```python
from build123d import *

# Parameters (mm, degrees)
BOSS_EXTRUDE1_DEPTH   = 2
BOSS_EXTRUDE1_2_DEPTH = 2
BOSS_EXTRUDE1_3_DEPTH = 2
SKETCH3_W             = 15
SKETCH3_H             = 6
BOSS_EXTRUDE2_DEPTH   = 2


with BuildPart() as part:
    # Sketch2 → Boss-Extrude1 (new body)
    with BuildSketch(Plane.XY):
        with BuildLine():
            Line((11.971746688, 19.734053644), (13.156348071, 19.734053669))
            ThreePointArc((13.156348071, 19.734053669), (13.179525443, 19.744291413), (13.193365664, 19.765515226))
            ThreePointArc((13.193365664, 19.765515226), (13.19739915, 19.821201025), (13.188063691, 19.8762467))
            ThreePointArc((13.188063691, 19.8762467), (13.111547426, 20.044582448), (13.014440765, 20.20194178))
            add(Edge.make_bspline(
                [(13.014440765, 20.20194178), (12.484950193, 21.013504257), (11.291530639, 21.013504258)],
                knots=[0.342748392, 0.342748392, 0.342748392, 1.381331673, 1.381331673, 1.381331673], degree=2, weights=[1, 0.868170932, 1]))
            Line((11.291530639, 21.013504258), (11.173022933, 21.013504277))
            add(Edge.make_bspline(
                [(11.173022933, 21.013504277), (9.165862366, 21.013504277), (9.16586234, 19.429763689)],
                knots=[4.81203319, 4.81203319, 4.81203319, 6.344970319, 6.344970319, 6.344970319], degree=2, weights=[1, 0.720364545, 1]))
            Line((9.16586234, 19.429763689), (9.165862348, 19.265041834))
            add(Edge.make_bspline(
                [(9.165862348, 19.265041834), (9.165862348, 17.681301204), (11.173022971, 17.681301277)],
                knots=[3.079807634, 3.079807634, 3.079807634, 4.612744788, 4.612744788, 4.612744788], degree=2, weights=[1, 0.720364536, 1]))
            Line((11.173022971, 17.681301277), (11.291530595, 17.681301231))
            add(Edge.make_bspline(
                [(11.291530595, 17.681301231), (12.48495018, 17.681301231), (13.014440765, 18.492863728)],
                knots=[1.760260959, 1.760260959, 1.760260959, 2.798844261, 2.798844261, 2.798844261], degree=2, weights=[1, 0.868170926, 1]))
            ThreePointArc((13.014440765, 18.492863728), (13.107795315, 18.64362681), (13.182053506, 18.804655688))
            ThreePointArc((13.182053506, 18.804655688), (13.196728173, 18.865824439), (13.194497656, 18.928689268))
            ThreePointArc((13.194497656, 18.928689268), (13.179302023, 18.955174053), (13.150618481, 18.965643321))
            Line((13.150618481, 18.965643321), (11.971746647, 18.965643321))
            ThreePointArc((11.971746647, 18.965643321), (11.923939268, 18.950452436), (11.893668965, 18.91045222))
            add(Edge.make_bspline(
                [(11.265198612, 18.440979368), (11.727360525, 18.440524679), (11.893668965, 18.91045222)],
                knots=[5.955155363, 5.955155363, 5.955155363, 7.020735544, 7.020735544, 7.020735544], degree=2, weights=[1, 0.86139323, 1]))
            add(Edge.make_bspline(
                [(11.189511072, 20.254442875), (10.402055714, 20.214623084), (10.44001251, 19.305183226), (10.477969307, 18.395743368), (11.265198612, 18.440979368)],
                knots=[3.181025595, 3.181025595, 3.181025595, 4.754799698, 4.754799698, 6.328573801, 6.328573801, 6.328573801], degree=2, weights=[1, 0.706053195, 1, 0.706053195, 1]))
            add(Edge.make_bspline(
                [(11.893668965, 19.789244771), (11.708556533, 20.312305593), (11.189511072, 20.254442875)],
                knots=[2.404042417, 2.404042417, 2.404042417, 3.565685694, 3.565685694, 3.565685694], degree=2, weights=[1, 0.83601209, 1]))
            ThreePointArc((11.893668965, 19.789244771), (11.923939288, 19.749244541), (11.971746688, 19.734053644))
        make_face()
    extrude(amount=BOSS_EXTRUDE1_DEPTH)



with BuildPart() as body_2:
    # Sketch2 → Boss-Extrude1 2 (new body)
    with BuildSketch(Plane.XY):
        with BuildLine():
            Line((7.784019348, 19.734053644), (8.968620799, 19.734053669))
            ThreePointArc((8.968620799, 19.734053669), (8.99179817, 19.744291413), (9.005638392, 19.765515226))
            ThreePointArc((9.005638392, 19.765515226), (9.009671877, 19.821201025), (9.000336418, 19.8762467))
            ThreePointArc((9.000336418, 19.8762467), (8.923820153, 20.044582448), (8.826713493, 20.20194178))
            add(Edge.make_bspline(
                [(8.826713493, 20.20194178), (8.29722292, 21.013504257), (7.103803365, 21.013504258)],
                knots=[0.342748392, 0.342748392, 0.342748392, 1.381331673, 1.381331673, 1.381331673], degree=2, weights=[1, 0.868170932, 1]))
            Line((7.103803365, 21.013504258), (6.98529566, 21.013504277))
            add(Edge.make_bspline(
                [(6.98529566, 21.013504277), (4.978135095, 21.013504277), (4.978135132, 19.429763689)],
                knots=[4.81203319, 4.81203319, 4.81203319, 6.344970317, 6.344970317, 6.344970317], degree=2, weights=[1, 0.720364545, 1]))
            Line((4.978135132, 19.429763689), (4.978135076, 19.265041834))
            add(Edge.make_bspline(
                [(4.978135076, 19.265041834), (4.978135076, 17.681301205), (6.985295697, 17.681301277)],
                knots=[3.079807634, 3.079807634, 3.079807634, 4.612744788, 4.612744788, 4.612744788], degree=2, weights=[1, 0.720364536, 1]))
            Line((6.985295697, 17.681301277), (7.103803322, 17.681301231))
            add(Edge.make_bspline(
                [(7.103803322, 17.681301231), (8.297222907, 17.681301231), (8.826713493, 18.492863728)],
                knots=[4.901853612, 4.901853612, 4.901853612, 5.940436915, 5.940436915, 5.940436915], degree=2, weights=[1, 0.868170926, 1]))
            ThreePointArc((8.826713493, 18.492863728), (8.920068042, 18.64362681), (8.994326233, 18.804655688))
            ThreePointArc((8.994326233, 18.804655688), (9.009000901, 18.865824439), (9.006770384, 18.928689268))
            ThreePointArc((9.006770384, 18.928689268), (8.99157475, 18.955174054), (8.962891207, 18.965643321))
            Line((8.962891207, 18.965643321), (7.784019375, 18.965643321))
            ThreePointArc((7.784019375, 18.965643321), (7.736211995, 18.950452436), (7.705941692, 18.91045222))
            add(Edge.make_bspline(
                [(7.07747134, 18.440979368), (7.539633252, 18.440524679), (7.705941692, 18.91045222)],
                knots=[5.955155363, 5.955155363, 5.955155363, 7.020735544, 7.020735544, 7.020735544], degree=2, weights=[1, 0.86139323, 1]))
            add(Edge.make_bspline(
                [(7.0017838, 20.254442875), (6.214328441, 20.214623084), (6.252285238, 19.305183226), (6.290242034, 18.395743368), (7.07747134, 18.440979368)],
                knots=[3.181025595, 3.181025595, 3.181025595, 4.754799698, 4.754799698, 6.328573801, 6.328573801, 6.328573801], degree=2, weights=[1, 0.706053195, 1, 0.706053195, 1]))
            add(Edge.make_bspline(
                [(7.705941692, 19.78924477), (7.520829261, 20.312305593), (7.0017838, 20.254442875)],
                knots=[2.404042417, 2.404042417, 2.404042417, 3.565685694, 3.565685694, 3.565685694], degree=2, weights=[1, 0.83601209, 1]))
            ThreePointArc((7.705941692, 19.78924477), (7.736211988, 19.74924456), (7.784019348, 19.734053644))
        make_face()
    extrude(amount=BOSS_EXTRUDE1_2_DEPTH)


with BuildPart() as body_3:
    # Sketch2 → Boss-Extrude1 3 (new body)
    with BuildSketch(Plane.XY):
        with BuildLine():
            Line((16.159473961, 19.734053644), (17.344075345, 19.734053669))
            ThreePointArc((17.344075345, 19.734053669), (17.367252716, 19.744291413), (17.381092938, 19.765515226))
            ThreePointArc((17.381092938, 19.765515226), (17.385126423, 19.821201025), (17.375790964, 19.8762467))
            ThreePointArc((17.375790964, 19.8762467), (17.2992747, 20.044582448), (17.202168039, 20.20194178))
            add(Edge.make_bspline(
                [(17.202168039, 20.20194178), (16.672677467, 21.013504257), (15.479257913, 21.013504258)],
                knots=[0.342748392, 0.342748392, 0.342748392, 1.381331673, 1.381331673, 1.381331673], degree=2, weights=[1, 0.868170932, 1]))
            Line((15.479257913, 21.013504258), (15.360750206, 21.013504277))
            add(Edge.make_bspline(
                [(15.360750206, 21.013504277), (13.353589639, 21.013504277), (13.353589613, 19.429763689)],
                knots=[4.81203319, 4.81203319, 4.81203319, 6.344970319, 6.344970319, 6.344970319], degree=2, weights=[1, 0.720364545, 1]))
            Line((13.353589613, 19.429763689), (13.353589622, 19.265041834))
            add(Edge.make_bspline(
                [(13.353589622, 19.265041834), (13.353589622, 17.681301204), (15.360750245, 17.681301277)],
                knots=[3.079807634, 3.079807634, 3.079807634, 4.612744788, 4.612744788, 4.612744788], degree=2, weights=[1, 0.720364536, 1]))
            Line((15.360750245, 17.681301277), (15.479257869, 17.681301231))
            add(Edge.make_bspline(
                [(15.479257869, 17.681301231), (16.672677453, 17.681301231), (17.202168039, 18.492863728)],
                knots=[1.760260959, 1.760260959, 1.760260959, 2.798844261, 2.798844261, 2.798844261], degree=2, weights=[1, 0.868170926, 1]))
            ThreePointArc((17.202168039, 18.492863728), (17.295522588, 18.64362681), (17.369780779, 18.804655688))
            ThreePointArc((17.369780779, 18.804655688), (17.384455447, 18.865824439), (17.38222493, 18.928689268))
            ThreePointArc((17.38222493, 18.928689268), (17.367029296, 18.955174053), (17.338345755, 18.965643321))
            Line((17.338345755, 18.965643321), (16.159473921, 18.965643321))
            ThreePointArc((16.159473921, 18.965643321), (16.111666541, 18.950452436), (16.081396238, 18.91045222))
            add(Edge.make_bspline(
                [(15.452925886, 18.440979368), (15.915087798, 18.440524679), (16.081396238, 18.91045222)],
                knots=[5.955155363, 5.955155363, 5.955155363, 7.020735544, 7.020735544, 7.020735544], degree=2, weights=[1, 0.86139323, 1]))
            add(Edge.make_bspline(
                [(15.377238346, 20.254442875), (14.589782987, 20.214623084), (14.627739784, 19.305183226), (14.665696581, 18.395743368), (15.452925886, 18.440979368)],
                knots=[3.181025595, 3.181025595, 3.181025595, 4.754799698, 4.754799698, 6.328573801, 6.328573801, 6.328573801], degree=2, weights=[1, 0.706053195, 1, 0.706053195, 1]))
            add(Edge.make_bspline(
                [(16.081396238, 19.789244771), (15.896283807, 20.312305593), (15.377238346, 20.254442875)],
                knots=[2.404042417, 2.404042417, 2.404042417, 3.565685694, 3.565685694, 3.565685694], degree=2, weights=[1, 0.83601209, 1]))
            ThreePointArc((16.081396238, 19.789244771), (16.111666561, 19.749244541), (16.159473961, 19.734053644))
        make_face()
    extrude(amount=BOSS_EXTRUDE1_3_DEPTH)


with BuildPart() as part_1:
    add(part.part)

    add(body_2.part)  # Boss-Extrude2 merges body 2

    add(body_3.part)  # Boss-Extrude2 merges body 3
    # Sketch3 → Boss-Extrude2 (add)
    with BuildSketch(Plane(origin=(0, 0, 0), x_dir=(-1, 0, 0), z_dir=(0, 0, -1))):
        with Locations((-11.178135076, 19.347504277)):
            Rectangle(SKETCH3_W, SKETCH3_H)
    extrude(amount=BOSS_EXTRUDE2_DEPTH)


solid = part_1.part
```
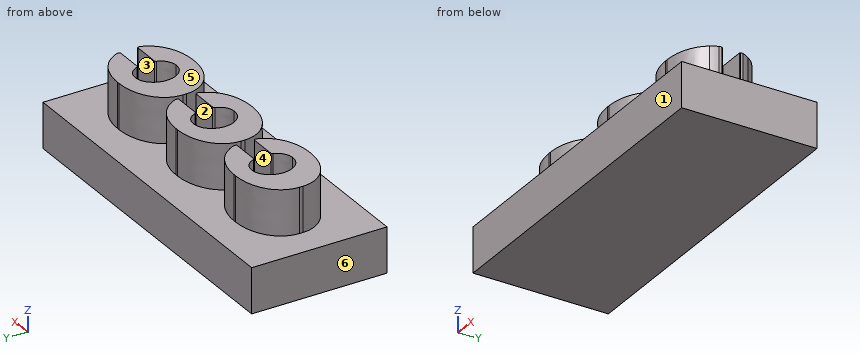
Read the model definition and answer for the solid it produces. Units are mm, in the model's axes. Face numbers are marked on the shaded views. A direction names the side the tool comes from. Round coordinates to 2 decimals unless told otherwise and drop trailing zeros. Write each loop counter-clockwise with the first axis right and the second up, starting at its lowest first coordinate (ties: lowest second). Pieces come first, ordered by that corner, then holes. Notation, with made-up numbers: (-27.75, -23) -> (-4.75, -23) arc R34 ccw to (-4.75, 14) -> close; hole circle Ø8 at (57, 81). An arc over 180 degrees is marked (long way). Answer in a Markdown table with one row per item. Add a question column.
1) Find section A-A, the plane y = 22. Determine the outline of the cut face in (x, z), and give its area (3 significant figures).
2) Find section C-C, the plane z = 0.85. State how many separate pieces and enclosed holes the cut face has, and give its area (3 significant figures).
3) Consider line 1 (X direction, y = 19.5, z = 1.1); line 2 (X direction, y = 20, z = 1.7); line 3 (Z direction, x = 15.25, y = 19). Determine where each line is inside the solid, lowest interval first.
4) Given P1, Ø0.6, axis at x = 8.5, z = 0.5, coming from the -Y side; P2, Ø0.6, axis at x = 17, z = 1.5, coming from the +Y side, each flat-ended and moving along its own axis, determine where each tip first touches the part or whether it passes through.
5) Determine the mould class of the marked faces 4, 5 and 6 for opening direction X: pulls with the +X half, pulls with the -X half, needs draft (parallel to the pull), parting line crosses it, or undercut.
6) Which of the six approach directions +Z, -Z, +X, -X, +Y, -Y give full straight-line access (tool end or side, diameter ignored) to the marked faces 1, 2 and 3?
7) Find section B-B, the plane x = 17.75. Determine the outline of the cut face in (y, z).
Findings below:
| question | item | result |
|---|---|---|
| 1 | outline | (3.68, -2) -> (18.68, -2) -> (18.68, 0) -> (3.68, 0) -> close |
| 1 | area | 30.0 mm² |
| 2 | separate pieces | 3 |
| 2 | enclosed holes | 0 |
| 2 | area | 23.3 mm² |
| 3 | line 1 | 4.98 to 6.26, 9.17 to 10.45, 13.36 to 14.64 |
| 3 | line 2 | 5.11 to 6.49, 7.59 to 8.95, 9.3 to 10.68, 11.78 to 13.13, 13.48 to 14.87, 15.97 to 17.32 |
| 3 | line 3 | -2 to 0 |
| 4 | P1 | y = 17.94 |
| 4 | P2 | y = 20.68 |
| 5 | face 4 | undercut |
| 5 | face 5 | needs draft |
| 5 | face 6 | pulls with the -X half |
| 6 | face 1 | +Z, -Z, +X, -X, -Y |
| 6 | face 2 | +Z |
| 6 | face 3 | +Z, +X |
| 7 | outline | (16.35, -2) -> (22.35, -2) -> (22.35, 0) -> (16.35, 0) -> close |
